Read the model definition and answer for the solid it produces. Units are mm, in the model's axes. Give positions to 0.01 mm unless a question says otherwise; leave off trailing zeros. Order: outer loops, then holes, each group sorted by start corner. A loop starts at its lowest first (then second) coordinate and runs counter-clockwise, first axis right, second up. Notation, with made-up numbers: (-23.75, -17) - (14.25, -17) arc R14 ccw to (14.25, -4) - close; hole circle Ø1 at (74.5, 20). An arc over 180 degrees is marked (long way). Use a Markdown table: item, result. Add a question column.
1. Consider L1, parallel to X at y = 0.75, z = 118; L2, parallel to Z at x = 411, y = 3.4; L3, parallel to X at y = 1.6, z = -85. Determine where each line is inside the solid, lowest interval first.
2. A cutting plane is placed at C-C on x = 671. Determine the outline of the cut face in (y, z), and give its area (3 significant figures).
3. Flat-ended cylindrical pins translate along their axes: P1, Ø4, axis at x = 426.27, z = -66.59, coming from the -Y side; P2, Ø2.5, axis at y = 1.5, z = -96, coming from the +X side. Find the tip coordinate at first contact, or state that the pin passes through.
4. A cutting plane is placed at A-A on y = 3.35. Determine the outline of the cut face in (x, z), and give its area (3 significant figures).
5. A cutting plane is placed at B-B on z = 135. Determine the outline of the cut face in (x, y).
```python
from build123d import *

# Parameters (mm, degrees)
RESSALTO_EXTRUS_O4_DEPTH = 5
ESBO_O2_R                = 2.5
CORTE_EXTRUS_O1_DEPTH    = 5


with BuildPart() as part:
    # Esboço1 → Ressalto-extrusão4 (new body)
    with BuildSketch(Plane(origin=(0, 0, 0), x_dir=(1, 0, 0), z_dir=(0, 1, 0))):
        with BuildLine():
            Line((516.267355398, -155.796995794), (396.267355398, -155.796995794))
            ThreePointArc((396.267355398, -155.796995794), (378.589685869, -148.474665324), (371.267355398, -130.796995794))
            Line((371.267355398, -130.796995794), (371.267355398, 81.588187759))
            Line((371.267355398, 81.588187759), (411.267355398, 81.588187759))
            Line((411.267355398, 81.588187759), (411.267355398, 121.588187759))
            Line((411.267355398, 121.588187759), (661.267355398, 121.588187759))
            Line((661.267355398, 121.588187759), (661.267355398, 81.588187759))
            Line((661.267355398, 81.588187759), (701.267355398, 81.588187759))
            Line((701.267355398, 81.588187759), (701.267355398, -130.796995794))
            ThreePointArc((701.267355398, -130.796995794), (693.945024928, -148.474665324), (676.267355398, -155.796995794))
            Line((676.267355398, -155.796995794), (556.267355398, -155.796995794))
            Line((556.267355398, -155.796995794), (556.267355398, -115.796995794))
            Line((556.267355398, -115.796995794), (516.267355398, -115.796995794))
            Line((516.267355398, -115.796995794), (516.267355398, -155.796995794))
        make_face()
    extrude(amount=RESSALTO_EXTRUS_O4_DEPTH)

    # Esboço2 → Corte-extrusão1 (cut)
    with BuildSketch(Plane(origin=(0, 5, 0), x_dir=(1, 0, 0), z_dir=(0, 1, 0))):
        with Locations(Location((571.267355398, -100.796995794, 0), (0, 0, 270))):
            Circle(ESBO_O2_R)
        with Locations(Location((501.267355398, -100.796995794, 0), (0, 0, 270))):
            Circle(ESBO_O2_R)
        with Locations(Location((646.267355398, 66.588187759, 0), (0, 0, 270))):
            Circle(ESBO_O2_R)
        with Locations(Location((426.267355398, 66.588187759, 0), (0, 0, 270))):
            Circle(ESBO_O2_R)
    extrude(amount=-CORTE_EXTRUS_O1_DEPTH, mode=Mode.SUBTRACT)


solid = part.part
```
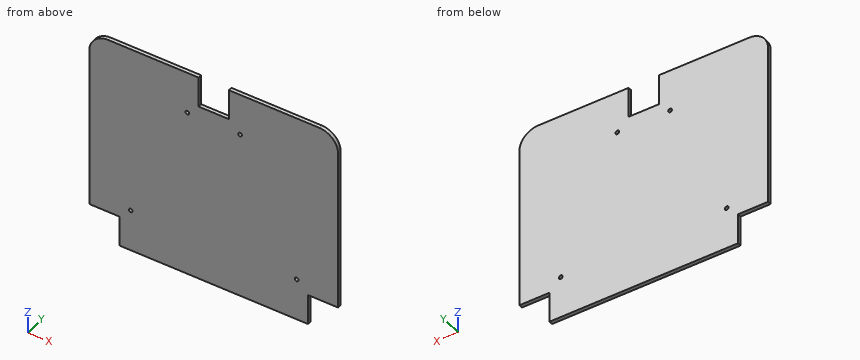
Output values:
| question | item | result |
|---|---|---|
| 1 | L1 | 371.27 to 516.27, 556.27 to 701.27 |
| 1 | L2 | -81.59 to 155.8 |
| 1 | L3 | 411.27 to 661.27 |
| 2 | outline | (0, -81.59) - (5, -81.59) - (5, 155.8) - (0, 155.8) - close |
| 2 | area | 1,190 mm² |
| 3 | P1 | through |
| 3 | P2 | x = 661.27 |
| 4 | outline | (371.27, -81.59) - (411.27, -81.59) - (411.27, -121.59) - (661.27, -121.59) - (661.27, -81.59) - (701.27, -81.59) - (701.27, 130.8) arc R25 ccw to (676.27, 155.8) - (556.27, 155.8) - (556.27, 115.8) - (516.27, 115.8) - (516.27, 155.8) - (396.27, 155.8) arc R25 ccw to (371.27, 130.8) - close; hole circle Ø5 at (426.27, -66.59); hole circle Ø5 at (501.27, 100.8); hole circle Ø5 at (571.27, 100.8); hole circle Ø5 at (646.27, -66.59) |
| 4 | area | 86,400 mm² |
| 5 | outline | (371.62, 0) - (516.27, 0) - (516.27, 5) - (371.62, 5) - close; (556.27, 0) - (700.91, 0) - (700.91, 5) - (556.27, 5) - close |
